For this review, take the finished solid that the model builds, in its own axes (mm). A direction names the side the tool comes from. Coordinates: 2 decimals unless noted, no trailing zeros. Write each loop counter-clockwise with the first axis right and the second up, starting at its lowest first coordinate (ties: lowest second). Pieces come first, ordered by that corner, then holes.
Autodesk Inventor part; units mm, degrees
ref_plane "YZ Plane" through (0, 0, 0) normal (1, 0, 0) x (0, 1, 0)
ref_plane "XZ Plane" through (0, 0, 0) normal (0, 1, 0) x (-1, 0, 0)
ref_plane "XY Plane" through (0, 0, 0) normal (0, 0, 1) x (1, 0, 0)
sketch "Skizze4" plane through (0, 0, 0) normal (0, 1, 0) x (-1, 0, 0)
  line L0 (-23.6102, 57) -> (23.6102, 57)
  line L1 (23.6102, 57) -> (57, 23.6102)
  line L2 (57, 23.6102) -> (57, -23.6102)
  line L3 (57, -23.6102) -> (23.6102, -57)
  line L4 (23.6102, -57) -> (-23.6102, -57)
  line L5 (-23.6102, -57) -> (-57, -23.6102)
  line L6 (-57, -23.6102) -> (-57, 23.6102)
  line L7 (-57, 23.6102) -> (-23.6102, 57)
  line L8 (79.8, 0) -> (-79.8, 0) construction
  line L9 (0, -79.8) -> (0, 79.8) construction
  circle A0 centre (-27, 27) radius 10
  circle A1 centre (-27, -27) radius 10
  circle A2 centre (27, -27) radius 10
  circle A3 centre (27, 27) radius 10
  point P0 (0, 0)
  point P1 (0, 0)
  dimension "d4" = 114
  dimension "d5" = 20
  dimension "d6" = 30
  dimension "d7" = 30
  dimension "d10" = 360
extrude "Extrusion2" add sketch "Skizze4" along normal blind 2.5
sketch "Skizze5" plane through (0, 0, 0) normal (0, -1, 0) x (1, 0, 0)
  circle A0 centre (-27, 27) radius 10 construction
  circle A1 centre (-27, -27) radius 10 construction
  circle A2 centre (27, -27) radius 10 construction
  circle A3 centre (27, 27) radius 10 construction
  line L0 (23.6102, 57) -> (-23.6102, 57) construction
  line L1 (-23.6102, 57) -> (-57, 23.6102) construction
  line L2 (-57, 23.6102) -> (-57, -23.6102) construction
  line L3 (-57, -23.6102) -> (-23.6102, -57) construction
  line L4 (-23.6102, -57) -> (23.6102, -57) construction
  line L5 (23.6102, -57) -> (57, -23.6102) construction
  line L6 (57, -23.6102) -> (57, 23.6102) construction
  line L7 (57, 23.6102) -> (23.6102, 57) construction
  line L8 (23.6102, 57) -> (57, 23.6102) construction
  line L9 (-57, -23.6102) -> (-57, 23.6102) construction
  line L10 (-23.6102, -57) -> (-57, -23.6102) construction
  line L11 (23.6102, -57) -> (-23.6102, -57) construction
  line L12 (57, 23.6102) -> (57, -23.6102) construction
  line L13 (-57, 17.1158) -> (-52.4078, 28.2024)
  line L14 (-57, 23.6102) -> (-23.6102, 57)
  line L15 (-57, 23.6102) -> (-57, -23.6102)
  line L16 (-57, 23.6102) -> (-52.4078, 28.2024)
  line L17 (-23.6102, 57) -> (-57, 23.6102)
  line L18 (-57, 23.6102) -> (-57, 17.1158)
  line L19 (-23.6102, -57) -> (-28.2024, -52.4078)
  line L20 (-17.1158, -57) -> (-28.2024, -52.4078)
  line L21 (-23.6102, -57) -> (-17.1158, -57)
  line L22 (57, -23.6102) -> (52.4078, -28.2024)
  line L23 (57, -17.1158) -> (52.4078, -28.2024)
  line L24 (57, -23.6102) -> (57, -17.1158)
  line L25 (23.6102, 57) -> (28.2024, 52.4078)
  line L26 (17.1158, 57) -> (28.2024, 52.4078)
  line L27 (23.6102, 57) -> (17.1158, 57)
  point P0 (0, 0)
  dimension "d21" = 22.5
  dimension "d22" = 12
  dimension "d25" = 360
extrude "Extrusion3" cut sketch "Skizze5" against normal blind 10
sketch "Skizze6" plane through (0, 2.5, 0) normal (0, 1, 0) x (1, 0, 0)
  line L0 (57, 17.1158) -> (52.4078, 28.2024)
  line L1 (52.4078, 28.2024) -> (23.6102, 57)
  line L2 (23.6102, 57) -> (-17.1158, 57)
  line L3 (-17.1158, 57) -> (-28.2024, 52.4078)
  line L4 (-28.2024, 52.4078) -> (-57, 23.6102)
  line L5 (-57, 23.6102) -> (-57, -17.1158)
  line L6 (-57, -17.1158) -> (-52.4078, -28.2024)
  line L7 (-52.4078, -28.2024) -> (-23.6102, -57)
  line L8 (-23.6102, -57) -> (17.1158, -57)
  line L9 (17.1158, -57) -> (28.2024, -52.4078)
  line L10 (28.2024, -52.4078) -> (57, -23.6102)
  line L11 (57, -23.6102) -> (57, 17.1158)
  circle A0 centre (-27, -27) radius 10
  circle A1 centre (-27, 27) radius 10
  circle A2 centre (27, 27) radius 10
  circle A3 centre (27, -27) radius 10
  point P0 (0, 0)
extrude "Extrusion4" cut sketch "Skizze6" against normal blind 1
sketch "Skizze7" plane through (0, 0, 0) normal (0, -1, 0) x (1, 0, 0)
  line L0 (52.4078, -28.2024) -> (57, -17.1158) construction
  line L1 (57, -17.1158) -> (57, 23.6102) construction
  line L2 (57, 23.6102) -> (28.2024, 52.4078) construction
  line L3 (28.2024, 52.4078) -> (17.1158, 57) construction
  line L4 (17.1158, 57) -> (-23.6102, 57) construction
  line L5 (-23.6102, 57) -> (-52.4078, 28.2024) construction
  line L6 (-52.4078, 28.2024) -> (-57, 17.1158) construction
  line L7 (-57, 17.1158) -> (-57, -23.6102) construction
  line L8 (-57, -23.6102) -> (-28.2024, -52.4078) construction
  line L9 (-28.2024, -52.4078) -> (-17.1158, -57) construction
  line L10 (-17.1158, -57) -> (23.6102, -57) construction
  line L11 (23.6102, -57) -> (52.4078, -28.2024) construction
  circle A0 centre (-27, 27) radius 10 construction
  circle A1 centre (-27, -27) radius 10 construction
  circle A2 centre (27, -27) radius 10 construction
  circle A3 centre (27, 27) radius 10 construction
  line L12 (-37, 27) -> (-37, -27)
  circle A4 centre (-27, -27) radius 10
  line L13 (-17, -27) -> (-17, 27)
  line L14 (37, -27) -> (37, 27)
  line L15 (17, -27) -> (17, 27)
  circle A5 centre (27, 27) radius 10
  arc A6 (-17, 27) -> (-37, 27) centre (-27, 27) ccw
  arc A7 (37, 27) -> (17, 27) centre (27, 27) ccw
  circle A8 centre (27, -27) radius 10
  arc A9 (17, -27) -> (37, -27) centre (27, -27) ccw
  circle A10 centre (-27, -27) radius 10
  arc A11 (-37, -27) -> (-17, -27) centre (-27, -27) ccw
  point P0 (0, 0)
extrude "Extrusion5" cut sketch "Skizze7" against normal through all
equation "\"d7\" = d6"
properties part number "Stage2" material "3.3547 AlMg4,5Mn (AW-5083/H111)"
1) For L1, parallel to X at y = 1.15, z = -13; L2, parallel to X at y = 1.35, z = 28; L3, parallel to Z at x = 35, y = 1, list the stretches that pass through material, from the lowest coordinate up.
2) The part is to be moulded in two halves that separate along X. For faces 3 (the face through (27, 1, -37)), 4 (the face through (-37.81, 0.74, 42.8)), 5 (the face through (37.81, 0.74, -42.8)), 6 (the face through (-27, 1, 37)), say which applies: pulls with the +X half, pulls with the -X half, needs draft (parallel to the pull), parting line crosses it, or undercut.
3) Consider section B-B (y = 0.4). Give the boundary of the cut face in (x, z), then the cut area to 3 significant figures.
4) Consider section A-A (z = 15). Give the boundary of the cut face in (x, y).
5) Consider section D-D (z = 46). Give the boundary of the cut face in (x, y).
6) Clearance check with a flat-ended pin moving along its axis: P1, Ø5, axis at x = 42, z = -21, coming from the -Y side. State where the tip first meets the part, or that it passes through.
7) Consider section C-C (z = 29.5). Give the boundary of the cut face in (x, y).
8) Tool access review of faces 1 (the face through (27, 1, 37)), 2 (the face through (54.736, 0.74, -22.581)): name each direction out of +Z, -Z, +X, -X, +Y, -Y from which nothing blocks a thin tool from reaching the whole face with its end or side.
Results:
1. L1: x = -57 to -37, -17 to 17, 37 to 57
1. L2: x = -52.49 to -36.95, -17.05 to 17.05, 36.95 to 52.61
1. L3: z = -45.61 to -33, 33 to 45.61
2. face 3: undercut
2. face 4: pulls with the -X half
2. face 5: pulls with the +X half
2. face 6: undercut
3. outline: (-57, -23.61) - (-28.2, -52.41) - (-17.12, -57) - (23.61, -57) - (52.41, -28.2) - (57, -17.12) - (57, 23.61) - (28.2, 52.41) - (17.12, 57) - (-23.61, 57) - (-52.41, 28.2) - (-57, 17.12) - close; hole (-37, -27) arc R10 ccw to (-17, -27) - (-17, 27) arc R10 ccw to (-37, 27) - close; hole (17, -27) arc R10 ccw to (37, -27) - (37, 27) arc R10 ccw to (17, 27) - close
3. area: 7,920 mm2
4. outline: (-57, 0) - (-37, 0) - (-37, 1.5) - (-57, 1.5) - close; (-17, 0) - (17, 0) - (17, 1.5) - (-17, 1.5) - close; (37, 0) - (57, 0) - (57, 1.5) - (37, 1.5) - close
5. outline: (-34.61, 0) - (34.61, 0) - (34.61, 1.5) - (-34.61, 1.5) - close
6. P1: stops at y = 0
7. outline: (-51.11, 0) - (-36.68, 0) - (-36.68, 1.5) - (-51.11, 1.5) - close; (-17.32, 0) - (17.32, 0) - (17.32, 1.5) - (-17.32, 1.5) - close; (36.68, 0) - (51.11, 0) - (51.11, 1.5) - (36.68, 1.5) - close
8. face 1: +Y, -Y
8. face 2: -Z, +X, +Y, -Y
